Input: dimensioned drawing with shaded views. Units: mm. Origin: part minimum x, y, z. A direction names the side the tool comes from. Give positions to 0.01 mm unless a question says otherwise; leave off trailing zeros. Write each loop counter-clockwise with the first axis right and the second up, starting at its lowest first coordinate (ties: lowest second). Pieces come first, ordered by that corner, then holes. Notation, with made-up numbers: (25, 28.25) -> (55, 28.25) arc R32 ccw to (55, 60.25) -> close; hole circle Ø11 at (-4, 12). An arc over 180 degrees is marked (long way). Answer as a JSON object with one key per item and string values. Group by question number.
(1) Material intervals for probe 1 along X at (y, z) = (6.8, 2.7); probe 2 along Y at (x, z) = (3, 2.4); probe 3 along Y at (x, z) = (0.8, 2.5), sorted ascending.
(2) Section query A-A on x = 1.6. Output: boundary loops of the cut face in (y, z), plus the area to 4 significant figures.
(3) Draft query along X for the marked faces 3, 4, 5 and 6. Return one class per face: +X half, -X half, draft (parallel to the pull), parting line (faces both ways), or undercut.
(4) Section query C-C on y = 1.5. Output: boundary loops of the cut face in (x, z), plus the area to 3 significant figures.
(5) Section query B-B on z = 2.05. Output: boundary loops of the cut face in (x, y), plus the area to 3 significant figures.
(6) Section query D-D on z = 0.5. Output: boundary loops of the cut face in (x, y), plus the area to 3 significant figures.
(7) Set-up query: the marked faces 1 and 2. Return all of +Z, -Z, +X, -X, +Y, -Y with unobstructed straight access to the full face (end or side cutting, diameter ignored); none if empty.
(8) Contact query for a flat-ended pin moving along its axis: pin 1 Ø1.5 at (x, z) = (2.5, 1.5) entering from -Y. Output: stop coordinate, or through.
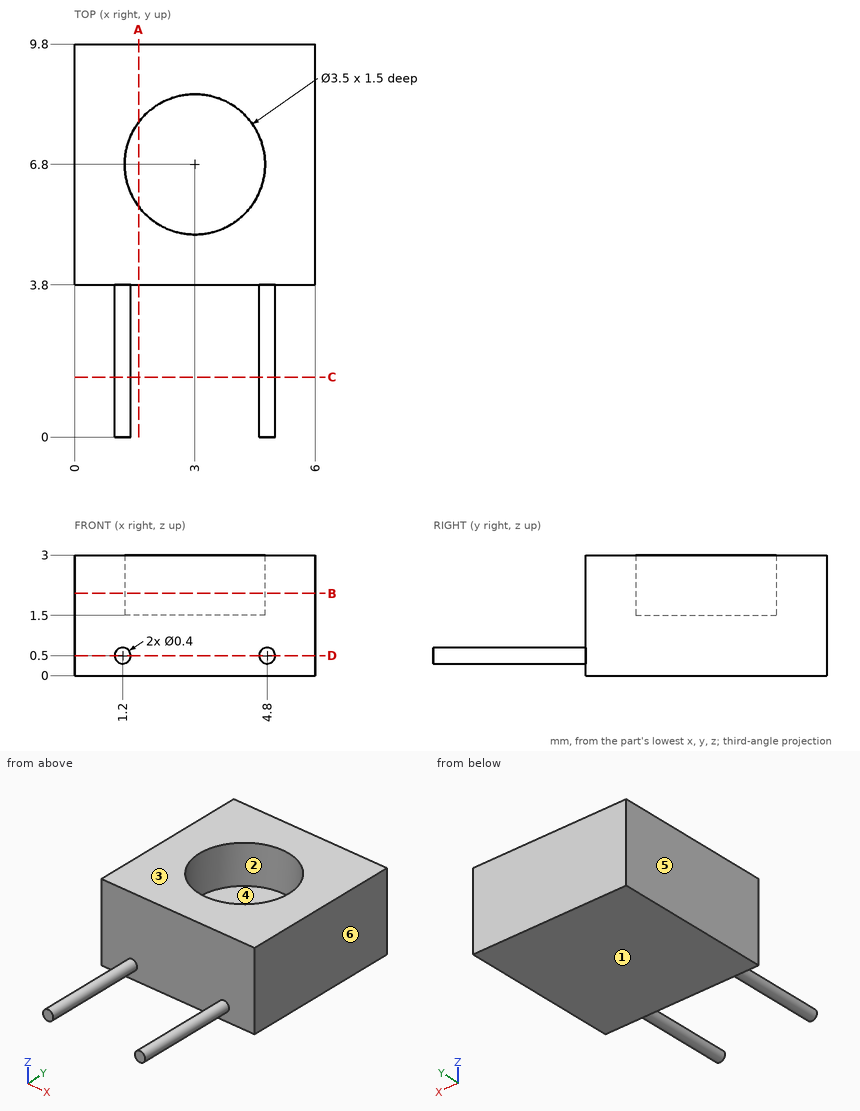
Answer list:
{
 "1": {"probe 1": "0 to 1.25, 4.75 to 6", "probe 2": "3.8 to 5.05, 8.55 to 9.8", "probe 3": "3.8 to 9.8"},
 "2": {"outline": "(3.8, 0) -> (9.8, 0) -> (9.8, 3) -> (7.85, 3) -> (7.85, 1.5) -> (5.75, 1.5) -> (5.75, 3) -> (3.8, 3) -> close", "area": "14.85 mm2"},
 "3": {"face 3": "draft", "face 4": "undercut", "face 5": "-X half", "face 6": "+X half"},
 "4": {"outline": "circle Ø0.4 at (1.2, 0.5); circle Ø0.4 at (4.8, 0.5)", "area": "0.251 mm2"},
 "5": {"outline": "(0, 3.8) -> (6, 3.8) -> (6, 9.8) -> (0, 9.8) -> close; hole circle Ø3.5 at (3, 6.8)", "area": "26.4 mm2"},
 "6": {"outline": "(0, 3.8) -> (1, 3.8) -> (1, 0) -> (1.4, 0) -> (1.4, 3.8) -> (4.6, 3.8) -> (4.6, 0) -> (5, 0) -> (5, 3.8) -> (6, 3.8) -> (6, 9.8) -> (0, 9.8) -> close", "area": "39.0 mm2"},
 "7": {"face 1": "-Z, +X, -X, +Y, -Y", "face 2": "+Z"},
 "8": {"pin 1": "y = 3.8"}
}
